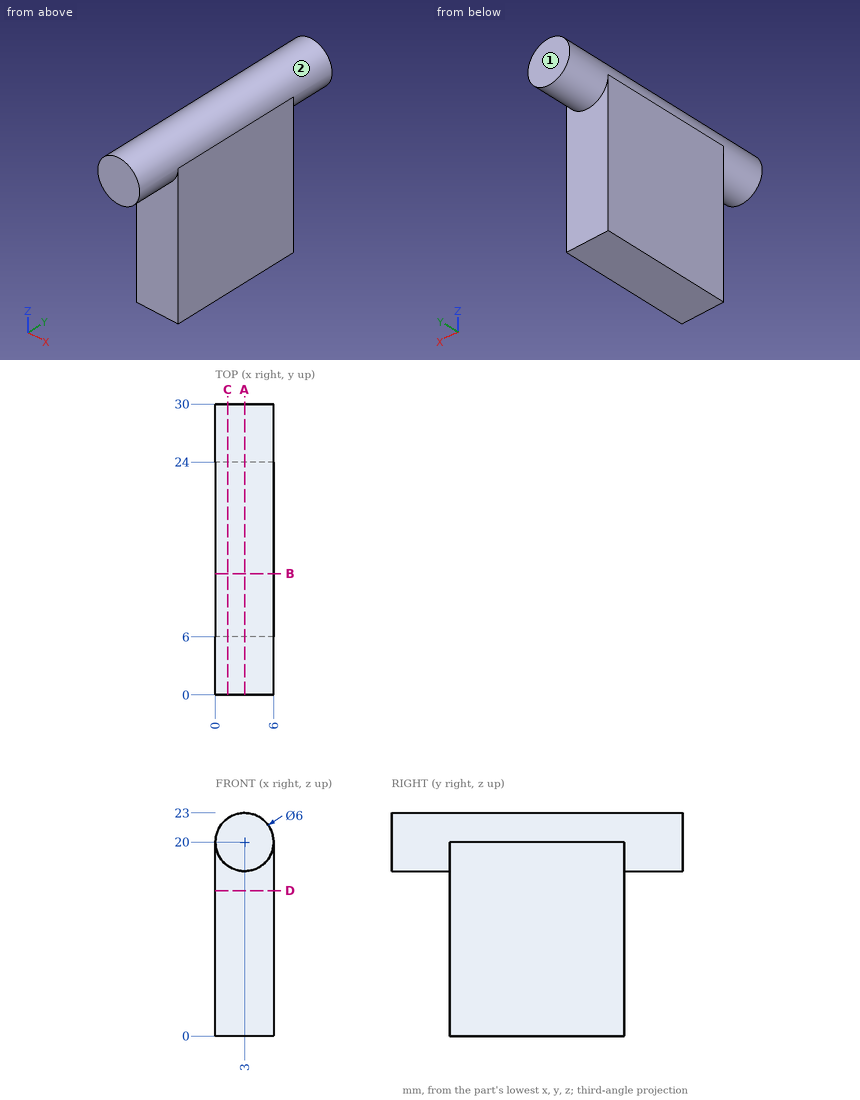
Here's the drawing with two shaded views (mm, measured from the low corner). I have some questions. A direction names the side the tool comes from. Coordinates: 2 decimals unless noted, no trailing zeros. Loops run counter-clockwise (first coordinate to the right, second up) from the corner with the lowest first, then second, coordinate; pieces in that order, holes last. Notation, with made-up numbers: (32.25, 80) -> (63.25, 80) arc R9 ccw to (63.25, 85) -> close; hole circle Ø10 at (-5, 6.25). An arc over 180 degrees is marked (long way). Put each result on its own line as item: value. Start each with the question number.
Q1. I want a section at D-D (z = 15). Write out the boundary of the cut face in (x, y).
Q2. I want a section at B-B (y = 12.5). Write out the boundary of the cut face in (x, z).
Q3. I want a section at A-A (x = 3). Write out the boundary of the cut face in (y, z), plus the area to 3 significant figures.
Q4. I'm going to push flat-ended pins straight in: P1, Ø1.8, axis at x = 3, z = 7, coming from the -Y side; P2, Ø3, axis at x = 4.5, y = 4.5, coming from the +Z side. Where does each tip first touch, or does it pass through?
Q5. If I drill on line 1 (Y direction, x = 5.75, z = 12.25); line 2 (Z direction, x = 5.25, y = 26); line 3 (Z direction, x = 2.75, y = 8), over which ranges is the centre line in solid material (lowest first)? Write a range as [from, to].
Q6. For the marked faces 1 and 2, which set-ups out of +Z, -Z, +X, -X, +Y, -Y let a thin tool reach every point of the face, with its end or its side?
Q7. I want a section at C-C (x = 1.25). Write out the boundary of the cut face in (y, z), plus the area to 3 significant figures.
Taken from the geometry:
1. outline: (0, 6) -> (6, 6) -> (6, 24) -> (0, 24) -> close
2. outline: (0, 0) -> (6, 0) -> (6, 19.97) arc R3 ccw (long way) to (0, 20) -> close
3. outline: (0, 17) -> (6, 17) -> (6, 0) -> (24, 0) -> (24, 17) -> (30, 17) -> (30, 23) -> (0, 23) -> close
3. area: 486 mm2
4. P1: stops at y = 6
4. P2: stops at z = 23
5. line 1: y = [6, 24]
5. line 2: z = [18.02, 21.98]
5. line 3: z = [0, 22.99]
6. face 1: +Z, -Z, +X, -X, +Y
6. face 2: none
7. outline: (0, 17.56) -> (6, 17.56) -> (6, 0) -> (24, 0) -> (24, 17.56) -> (30, 17.56) -> (30, 22.44) -> (0, 22.44) -> close
7. area: 462 mm2
